Read the model definition and answer for the solid it produces. Units are mm, in the model's axes. A direction names the side the tool comes from. Give positions to 0.01 mm unless a question says otherwise; leave off trailing zeros. Loops run counter-clockwise (first coordinate to the right, second up) from the corner with the lowest first, then second, coordinate; pieces in that order, holes last. Notation, with made-up numbers: (-17, 63) - (42, 63) arc R10 ccw to (42, 74) - close; hole circle Ø10 at (-11.5, -2). An arc over 180 degrees is marked (long way). Write each question's results on one line, items separated by ' | '. Start each with the question number.
Q1. The part is cut by section B-B, the plane z = -73.5. Write down the section's boundary in (x, y) (3 decimals), plus the area to 3 significant figures.
Q2. Find the intervals of material crossed by line 1 (Y direction, x = -4.5, z = -76); line 2 (Z direction, x = -2, y = -1); line 3 (X direction, y = -0.25, z = -74.5) (3 decimals), in increasing order. Write a range as from..to.
Q3. For faces 1 (the flat face through (-2, -4, -69.85)), 2 (the cylindrical face through (-0.11, 0.63, 5.08)), determine the directions among +Z, -Z, +X, -X, +Y, -Y from which every point of the face is accessible in a straight line to the end or side of a thin tool.
Q4. Given pin 1 (3 mm diameter, centred on x = -1.5, y = -4.5, fed in from +Z); pin 2 (3 mm diameter, centred on x = -1.5, z = -35, fed in from -Y), each flat-ended and moving along its own axis, determine where each tip first touches the part or whether it passes through.
Q5. The part is cut by section C-C, the plane z = -46.5. Write down the section's boundary in (x, y), plus the area to 3 significant figures.
Q6. The part is cut by section A-A, the plane x = 0. Write down the section's boundary in (y, z) (3 decimals), plus the area to 3 significant figures.
Q7. Determine the mould class of faces 3 (the flat face through (0, 1.27, -39)), 4 (the cylindrical face through (-1.62, 0.63, -2.12)), 5 (the flat face through (1.905, -5, -76)) for opening direction X: +X half, -X half, draft (parallel to the pull), parting line (faces both ways), or undercut.
```python
from build123d import *

# Parameters (mm, degrees)
SKETCH1_R           = 5.08
SKETCH1_R_2         = 2.667
BOSS_EXTRUDE1_DEPTH = 1.27
BOSS_EXTRUDE5_DEPTH = 1.27
SKETCH6_W           = 6.985
SKETCH6_H           = 12.7
BOSS_EXTRUDE6_DEPTH = 7.62
CUT_EXTRUDE2_REACH  = 85.195
SKETCH7_R           = 1.27


with BuildPart() as part:
    # Sketch1 → Boss-Extrude1 (new body)
    with BuildSketch(Plane(origin=(0, 0, 0), x_dir=(1, 0, 0), z_dir=(0, 1, 0))):
        with Locations(Location((0, 0, 0), (0, 0, 270))):
            Circle(SKETCH1_R)
        with Locations(Location((0, 0, 0), (0, 0, 270))):
            Circle(SKETCH1_R_2, mode=Mode.SUBTRACT)
    extrude(amount=BOSS_EXTRUDE1_DEPTH)

    # Sketch5 → Boss-Extrude5 (add)
    with BuildSketch(Plane(origin=(0, 0, 0), x_dir=(-1, 0, 0), z_dir=(0, -1, 0))):
        with BuildLine():
            Line((-5.08, 0), (-5.08, 82.55))
            Line((-5.08, 82.55), (5.08, 82.55))
            Line((5.08, 82.55), (5.08, 0))
            ThreePointArc((5.08, 0), (0, 5.08), (-5.08, 0))
        make_face()
    extrude(amount=-BOSS_EXTRUDE5_DEPTH)

    # Sketch6 → Boss-Extrude6 (add)
    with BuildSketch(Plane.XZ):
        with Locations((-1.5875, -76.2)):
            Rectangle(SKETCH6_W, SKETCH6_H)
    extrude(amount=BOSS_EXTRUDE6_DEPTH)

    # Sketch7 → Cut-Extrude2 (cut, up to next)
    with BuildSketch(Plane(origin=(1.905, 0, 0), x_dir=(0, 0, -1), z_dir=(1, 0, 0)), mode=Mode.PRIVATE) as cut_extrude2_sk1:
        with Locations((76.157654901, -3.175)):
            Circle(SKETCH7_R)
    cut_extrude2_tool1 = extrude(cut_extrude2_sk1.sketch, amount=-CUT_EXTRUDE2_REACH, mode=Mode.PRIVATE) & part.part
    add(cut_extrude2_tool1.solids().sort_by_distance((1.905, -3.175, -76.157655))[0], mode=Mode.SUBTRACT)


solid = part.part
```
Check sheet entries:
1) outline: (-5.08, -7.62) - (1.905, -7.62) - (1.905, 0) - (5.08, 0) - (5.08, 1.27) - (-5.08, 1.27) - close | area: 66.1 mm^2
2) line 1: y = -7.62..-4.44, -1.91..1.27 | line 2: z = -82.55..-69.85 | line 3: x = -5.08..1.905
3) face 1: +Z, +X, -X, -Y | face 2: +Z, +Y, -Y
4) pin 1: stops at z = -69.85 | pin 2: stops at y = 0
5) outline: (-5.08, 0) - (5.08, 0) - (5.08, 1.27) - (-5.08, 1.27) - close | area: 12.9 mm^2
6) outline: (-7.62, -82.55) - (1.27, -82.55) - (1.27, -2.667) - (0, -2.667) - (0, -69.85) - (-7.62, -69.85) - close; (0, 2.667) - (1.27, 2.667) - (1.27, 5.08) - (0, 5.08) - close; hole circle Ø2.54 at (-3.175, -76.158) | area: 196 mm^2
7) face 3: draft | face 4: undercut | face 5: +X half
